Geometry check sheet. Reference: the model listing, model coordinates, mm. A direction names the side the tool comes from. Coordinates: 2 decimals unless noted, no trailing zeros. Order: outer loops, then holes, each group sorted by start corner. A loop starts at its lowest first (then second) coordinate and runs counter-clockwise, first axis right, second up. Notation, with made-up numbers: (7, -39) -> (59, -39) arc R24 ccw to (59, -28) -> close; hole circle Ø3 at (-8.5, 84.5). An arc over 180 degrees is marked (long way). Answer as CSV lines item,"result". Start each with the question number.
from build123d import *

# Parameters (mm, degrees)
SKETCH_R        = 55
SKETCH_R_2      = 12.5
SKETCH_R_3      = 1.5
PAD_DEPTH       = 3
SKETCH001_R     = 20
SKETCH001_R_2   = 12.5
PAD001_DEPTH    = 8
SKETCH002_R     = 20
SKETCH002_R_2   = 4
PAD002_DEPTH    = 4
SKETCH003_R     = 8
SKETCH003_R_2   = 4
PAD003_DEPTH    = 6
CHAMFER_SIZE    = 2
CHAMFER001_SIZE = 2
CHAMFER002_SIZE = 2
CHAMFER003_SIZE = 1
CHAMFER004_SIZE = 1


with BuildPart() as part:
    # Sketch → Pad (new body)
    with BuildSketch(Plane.XY):
        Circle(SKETCH_R)
        Circle(SKETCH_R_2, mode=Mode.SUBTRACT)
        with Locations((35.355339, 35.355339)):
            Circle(SKETCH_R_3, mode=Mode.SUBTRACT)
        with Locations((-35.355339, 35.355339)):
            Circle(SKETCH_R_3, mode=Mode.SUBTRACT)
        with Locations((-35.355339, -35.355339)):
            Circle(SKETCH_R_3, mode=Mode.SUBTRACT)
        with Locations((35.355339, -35.355339)):
            Circle(SKETCH_R_3, mode=Mode.SUBTRACT)
    extrude(amount=PAD_DEPTH)

    # Sketch001 (on Face8 of Pad) → Pad001 (join)
    with BuildSketch(Plane.XY.offset(3)):
        Circle(SKETCH001_R)
        Circle(SKETCH001_R_2, mode=Mode.SUBTRACT)
    extrude(amount=PAD001_DEPTH)

    # Sketch002 (on Face11 of Pad001) → Pad002 (join)
    with BuildSketch(Plane.XY.offset(11)):
        Circle(SKETCH002_R)
        Circle(SKETCH002_R_2, mode=Mode.SUBTRACT)
    extrude(amount=PAD002_DEPTH)

    # Sketch003 (on Face13 of Pad002) → Pad003 (join)
    with BuildSketch(Plane.XY.offset(15)):
        Circle(SKETCH003_R)
        Circle(SKETCH003_R_2, mode=Mode.SUBTRACT)
    extrude(amount=PAD003_DEPTH)

    # Sketch004 → Revolution (revolve)
    with BuildSketch(Plane.XZ):
        Polygon((25, 3), (20, 8), (20, 3), align=None)
    revolve(axis=Axis((0, 0, 0), (0, 0, 1)))

    # Chamfer
    chamfer_edges = [part.edges().sort_by_distance(p)[0] for p in [
        (-20, 0, 15),
    ]]
    chamfer(chamfer_edges, length=CHAMFER_SIZE)

    # Chamfer001
    chamfer001_edges = [part.edges().sort_by_distance(p)[0] for p in [
        (-8, 0, 21),
    ]]
    chamfer(chamfer001_edges, length=CHAMFER001_SIZE)

    # Chamfer002
    chamfer002_edges = [part.edges().sort_by_distance(p)[0] for p in [
        (-12.5, 0, 0),
    ]]
    chamfer(chamfer002_edges, length=CHAMFER002_SIZE)

    # Chamfer003
    chamfer003_edges = [part.edges().sort_by_distance(p)[0] for p in [
        (-4, 0, 11),
    ]]
    chamfer(chamfer003_edges, length=CHAMFER003_SIZE)

    # Chamfer004
    chamfer004_edges = [part.edges().sort_by_distance(p)[0] for p in [
        (-4, 0, 21),
    ]]
    chamfer(chamfer004_edges, length=CHAMFER004_SIZE)


solid = part.part
Q1. Sectioned sample at C-C, the plane z = 5.5. Record the cut outline in (x, y).
Q2. Go/stop test with flat-tipped pins: pin 1 Ø3.5 at (x, y) = (-35.36, 35.36) entering from +Z; pin 2 Ø5 at (x, z) = (-33, 4.5) entering from +Y; pin 3 Ø2 at (y, z) = (14, 9) entering from -X. Record where each tip stops, or that it passes through.
Q3. Access from +Z, -Z, +X, -X, +Y, -Y to the whole of each face (thin tool, end or side, straight path). Record for faces 1 (the flat face through (4, -8, 15)), 2 (the flat face through (-0.2, -5.4, 11)), 3 (the flat face through (11, -11, 0)).
Q4. Sectioned sample at D-D, the plane x = 44. Record the cut outline in (y, z), then the cut area to 3 significant figures.
Q5. Thickness scan on L1, parallel to Y at x = 0, z = 17; L2, parallel to Z at x = 33, y = -26.5; L3, parallel to Z at x = 9, y = 13. Record the ranges inside material, lowest first.
Geometry results:
1,outline,"circle Ø45 at (0, 0); hole circle Ø25 at (0, 0)"
2,pin 1,"stops at z = 3"
2,pin 2,"stops at y = 45.43"
2,pin 3,"stops at x = -15.2"
3,face 1,"+Z"
3,face 2,"-Z"
3,face 3,"-Z, +X, -X, +Y, -Y"
4,outline,"(-33, 0) -> (33, 0) -> (33, 3) -> (-33, 3) -> close"
4,area,"198 mm^2"
5,L1,"y = -8 to -4, 4 to 8"
5,L2,"z = 0 to 3"
5,L3,"z = 0 to 15"
